Design review of the part built by this model. Coordinates are the model's own, in mm. Coordinates: 2 decimals unless noted, no trailing zeros. Write each loop counter-clockwise with the first axis right and the second up, starting at its lowest first coordinate (ties: lowest second). Pieces come first, ordered by that corner, then holes. Notation, with made-up numbers: (-18, 58) -> (-7, 58) arc R16 cw to (-7, 63) -> close; hole circle Ø2 at (83, -19). An arc over 180 degrees is marked (long way). Return JSON: item names as keys, results as strings. Group by question number.
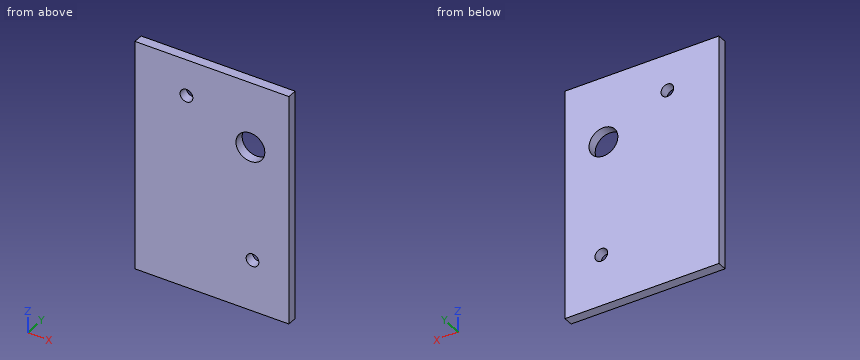
from build123d import *

# Parameters (mm, degrees)
SKETCH1_W           = 50.8
SKETCH1_H           = 76.2
BOSS_EXTRUDE1_DEPTH = 3.175
SKETCH2_R           = 4.7625
CUT_EXTRUDE1_DEPTH  = 4.175
SKETCH3_R           = 2.1
CUT_EXTRUDE2_DEPTH  = 4.175


with BuildPart() as part:
    # Sketch1 → Boss-Extrude1 (new body)
    with BuildSketch(Plane(origin=(0, 0, 0), x_dir=(1, 0, 0), z_dir=(0, 1, 0))):
        Rectangle(SKETCH1_W, SKETCH1_H)
    extrude(amount=BOSS_EXTRUDE1_DEPTH)

    # Sketch2 → Cut-Extrude1 (cut, through all)
    with BuildSketch(Plane(origin=(0, 3.175, 0), x_dir=(1, 0, 0), z_dir=(0, 1, 0))):
        with Locations((12.7, -16.51)):
            Circle(SKETCH2_R)
    extrude(amount=-CUT_EXTRUDE1_DEPTH, mode=Mode.SUBTRACT)

    # Sketch3 → Cut-Extrude2 (cut, through all)
    with BuildSketch(Plane(origin=(0, 3.175, 0), x_dir=(1, 0, 0), z_dir=(0, 1, 0))):
        with Locations((13.4, 21.1)):
            Circle(SKETCH3_R)
        with Locations((-8.4, -26.1)):
            Circle(SKETCH3_R)
    extrude(amount=-CUT_EXTRUDE2_DEPTH, mode=Mode.SUBTRACT)


solid = part.part
Q1. Wall thickness on L1, parallel to X at y = 1, z = 16.51; L2, parallel to X at y = 1.4, z = 26.1; L3, parallel to Z at x = 13.4, y = 0.8: over which ranges is each line inside the solid? List them lowest first.
Q2. We need section B-B on y = 1.25. Write out the cut boundary in (x, z) (1 decimal).
Q3. We need section A-A on z = 16.51. Write out the cut boundary in (x, y) (1 decimal).
Q4. We need section C-C on z = -21.1. Write out the cut boundary in (x, y) (3 decimals), plus the area to 3 significant figures.
Q5. For P1, Ø3.5, axis at x = -8.4, z = 26.1, coming from the +Y side, flat-tipped, find the tip position at first contact; note if it passes through.
Findings below:
{
 "1": {"L1": "x = -25.4 to 7.94, 17.46 to 25.4", "L2": "x = -25.4 to -10.5, -6.3 to 25.4", "L3": "z = -38.1 to -23.2, -19 to 11.8, 21.22 to 38.1"},
 "2": {"outline": "(-25.4, -38.1) -> (25.4, -38.1) -> (25.4, 38.1) -> (-25.4, 38.1) -> close; hole circle Ø4.2 at (-8.4, 26.1); hole circle Ø9.5 at (12.7, 16.5); hole circle Ø4.2 at (13.4, -21.1)"},
 "3": {"outline": "(-25.4, 0) -> (7.9, 0) -> (7.9, 3.2) -> (-25.4, 3.2) -> close; (17.5, 0) -> (25.4, 0) -> (25.4, 3.2) -> (17.5, 3.2) -> close"},
 "4": {"outline": "(-25.4, 0) -> (11.3, 0) -> (11.3, 3.175) -> (-25.4, 3.175) -> close; (15.5, 0) -> (25.4, 0) -> (25.4, 3.175) -> (15.5, 3.175) -> close", "area": "148 mm^2"},
 "5": {"P1": "passes through"}
}
